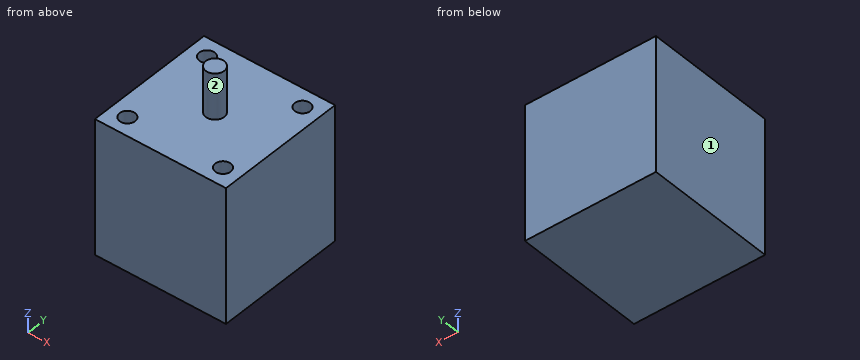
```python
from build123d import *

# Parameters (mm, degrees)
SKETCH1_W           = 42.5
SKETCH1_H           = 42.5
BOSS_EXTRUDE1_DEPTH = 43.75
SKETCH2_R           = 2.5
CUT_EXTRUDE1_DEPTH  = 5
SKETCH3_R           = 3
BOSS_EXTRUDE2_DEPTH = 14.86


with BuildPart() as part:
    # Sketch1 → Boss-Extrude1 (new body)
    with BuildSketch(Plane.XY):
        Rectangle(SKETCH1_W, SKETCH1_H)
    extrude(amount=BOSS_EXTRUDE1_DEPTH)

    # Sketch2 → Cut-Extrude1 (cut)
    with BuildSketch(Plane.XY.offset(43.75)):
        with Locations((-15.495, 15.495)):
            Circle(SKETCH2_R)
        with Locations((15.495, 15.495)):
            Circle(SKETCH2_R)
        with Locations((15.495, -15.495)):
            Circle(SKETCH2_R)
        with Locations((-15.495, -15.495)):
            Circle(SKETCH2_R)
    extrude(amount=-CUT_EXTRUDE1_DEPTH, mode=Mode.SUBTRACT)

    # Sketch3 → Boss-Extrude2 (add)
    with BuildSketch(Plane.XY.offset(43.75)):
        Circle(SKETCH3_R)
    extrude(amount=BOSS_EXTRUDE2_DEPTH)


solid = part.part
```
Could you check a few things on this model? Use its own coordinates, in mm. Face numbers are marked on the shaded views. A direction names the side the tool comes from. Round coordinates to 2 decimals unless told otherwise and drop trailing zeros. Write each loop counter-clockwise with the first axis right and the second up, starting at its lowest first coordinate (ties: lowest second). Pieces come first, ordered by that corner, then holes.
(1) If I drill on probe 1 along X at (y, z) = (16.5, 41); probe 2 along Y at (x, z) = (14.5, 41); probe 3 along Z at (x, y) = (1.5, 6), over which ranges is the centre line in solid material (lowest first)?
Findings below:
probe 1: x = -21.25 to -17.78, -13.21 to 13.21, 17.78 to 21.25
probe 2: y = -21.25 to -17.79, -13.2 to 13.2, 17.79 to 21.25
probe 3: z = 0 to 43.75
(2) Suppose I cut it at A-A on x = 0. Write out the boundary of the cut face in (y, z).
Findings below:
outline: (-21.25, 0) - (21.25, 0) - (21.25, 43.75) - (3, 43.75) - (3, 58.61) - (-3, 58.61) - (-3, 43.75) - (-21.25, 43.75) - close
(3) Which directions (+Z, -Z, +X, -X, +Y, -Y) give clear straight access to the entire face, cutting with the end or side of a thin tool? Please do the marked faces 1 and 2.
Findings below:
face 1: +Z, -Z, -X, +Y, -Y
face 2: +Z
(4) Suppose I cut it at C-C on y = 9. Write out the boundary of the cut face in (x, z), and give its area (3 significant figures).
Findings below:
outline: (-21.25, 0) - (21.25, 0) - (21.25, 43.75) - (-21.25, 43.75) - close
area: 1,860 mm2
(5) For pin 1 (3 mm diameter, centred on x = 15.495, y = -15.495, fed in from -Z); pin 2 (12 mm diameter, centred on x = -14, y = 2, fed in from +Z); pin 3 (1.5 mm diameter, centred on x = -16.5, y = 15, fed in from +Z), each with a flat end and sliding along its axis, tell me the tip position at first contact or that it passes through.
Findings below:
pin 1: stops at z = 0
pin 2: stops at z = 43.75
pin 3: stops at z = 38.75
